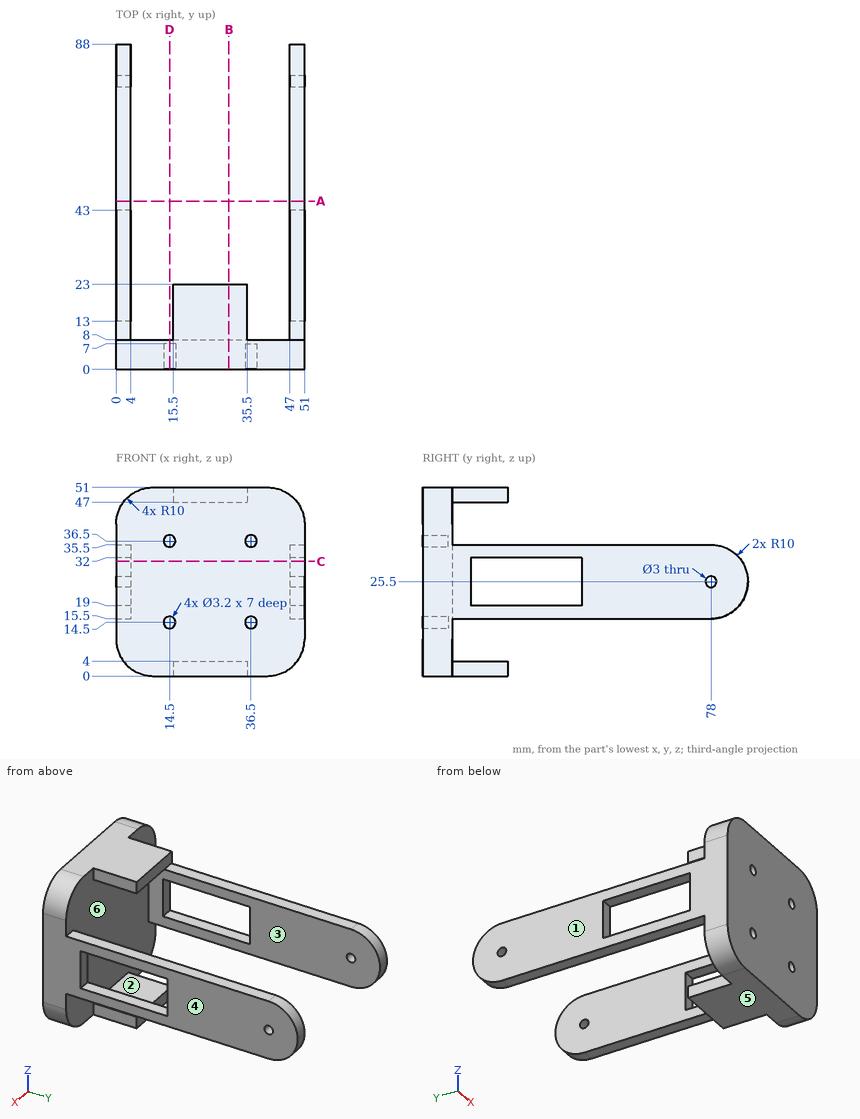
Could you check a few things on this drawing? It's one solid part, dimensions in mm from its lowest x, y, z. A direction names the side the tool comes from. Give positions to 0.01 mm unless a question says otherwise; leave off trailing zeros. Write each loop counter-clockwise with the first axis right and the second up, starting at its lowest first coordinate (ties: lowest second). Pieces come first, ordered by that corner, then holes. Notation, with made-up numbers: (-12.5, 48) -> (13.5, 48) arc R21 ccw to (13.5, 85) -> close; hole circle Ø11 at (-30, -2). An arc over 180 degrees is marked (long way). Answer as CSV lines item,"result". Start each with the question number.
(1) If we section it at C-C, the plane z = 31: Write out the boundary of the cut face in (x, y), and give its area (3 significant figures).
(2) If we mould it in two halves opening along X, with no side actions, what happens to the marked faces 4, 5 and 6? For each: +X half, -X half, draft (parallel to the pull), parting line (faces both ways), or undercut.
(3) If we section it at B-B, the plane x = 30.5: Write out the boundary of the cut face in (y, z).
(4) Please list where these lines run through material, in increasing order: line 1 (X direction, y = 3, z = 14.5); line 2 (Y direction, x = 1.45, z = 25.5); line 3 (Z direction, x = 49.2, y = 78).
(5) If we section it at A-A, the plane y = 45.5: Write out the boundary of the cut face in (x, z).
(6) I'm going to push flat-ended pins straight in: pin 1 Ø1.6 at (x, z) = (14.5, 37) entering from -Y; pin 2 Ø4.5 at (y, z) = (19, 2.5) entering from -X; pin 3 Ø2.5 at (x, z) = (36.5, 36.5) entering from +Y. Where does each tip first touch, or does it pass through?
(7) If we section it at D-D, the plane x = 14.5: Write out the boundary of the cut face in (y, z).
(8) Which directions (+Z, -Z, +X, -X, +Y, -Y) give clear straight access to the entire face, cutting with the end or side of a thin tool? Please do the marked faces 1, 2 and 3.
Answer list:
1,outline,"(0, 0) -> (51, 0) -> (51, 13) -> (47, 13) -> (47, 8) -> (4, 8) -> (4, 13) -> (0, 13) -> close; (0, 43) -> (4, 43) -> (4, 86.35) -> (0, 86.35) -> close; (47, 43) -> (51, 43) -> (51, 86.35) -> (47, 86.35) -> close"
1,area,"795 mm^2"
2,face 4,"+X half"
2,face 5,"draft"
2,face 6,"undercut"
3,outline,"(0, 0) -> (23, 0) -> (23, 4) -> (8, 4) -> (8, 47) -> (23, 47) -> (23, 51) -> (0, 51) -> close"
4,line 1,"0 to 12.9, 16.1 to 34.9, 38.1 to 51"
4,line 2,"0 to 13, 43 to 76.5, 79.5 to 88"
4,line 3,"15.5 to 24, 27 to 35.5"
5,outline,"(0, 15.5) -> (4, 15.5) -> (4, 35.5) -> (0, 35.5) -> close; (47, 15.5) -> (51, 15.5) -> (51, 35.5) -> (47, 35.5) -> close"
6,pin 1,"y = 7"
6,pin 2,"x = 15.5"
6,pin 3,"y = 8"
7,outline,"(0, 0) -> (8, 0) -> (8, 51) -> (0, 51) -> (0, 38.1) -> (7, 38.1) -> (7, 34.9) -> (0, 34.9) -> (0, 16.1) -> (7, 16.1) -> (7, 12.9) -> (0, 12.9) -> close"
8,face 1,"+Z, -Z, -X, +Y, -Y"
8,face 2,"+X, -X, +Y"
8,face 3,"+Z, -Z, +Y"
